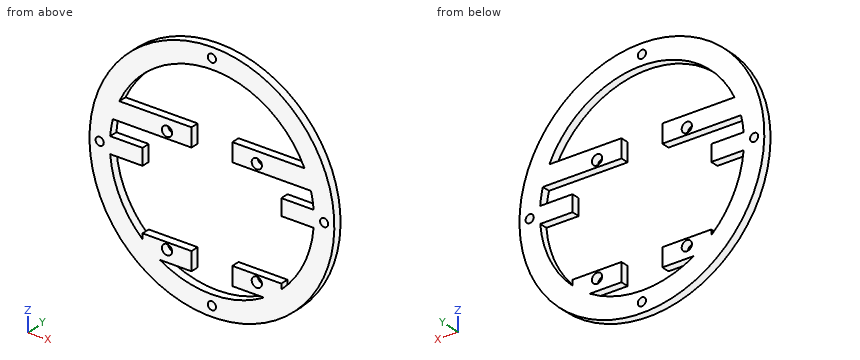
```python
from build123d import *

# Parameters (mm, degrees)
SKETCH1_R           = 30
SKETCH1_R_2         = 25
BOSS_EXTRUDE1_DEPTH = 2
SKETCH2_R           = 1
CUT_EXTRUDE1_DEPTH  = 43.473521163
BOSS_EXTRUDE2_DEPTH = 2
BOSS_EXTRUDE3_DEPTH = 2
CUT_EXTRUDE2_DEPTH  = 2
BOSS_EXTRUDE4_DEPTH = 2
SKETCH16_R          = 1.25
CUT_EXTRUDE3_DEPTH  = 2


with BuildPart() as part:
    # Sketch1 → Boss-Extrude1 (new body)
    with BuildSketch(Plane(origin=(0, 0, 0), x_dir=(1, 0, 0), z_dir=(0, 1, 0))):
        with Locations(Location((0, 0, 0), (0, 0, 270))):
            Circle(SKETCH1_R)
        with Locations(Location((0, 0, 0), (0, 0, 270))):
            Circle(SKETCH1_R_2, mode=Mode.SUBTRACT)
    extrude(amount=BOSS_EXTRUDE1_DEPTH)

    # Sketch2 → Cut-Extrude1 (cut, through all)
    with BuildSketch(Plane(origin=(0, 2, 0), x_dir=(1, 0, 0), z_dir=(0, 1, 0))):
        with Locations(Location((0, 27.5, 0), (0, 0, 270))):
            Circle(SKETCH2_R)
        with Locations(Location((27.5, 0, 0), (0, 0, 270))):
            Circle(SKETCH2_R)
        with Locations(Location((0, -27.5, 0), (0, 0, 270))):
            Circle(SKETCH2_R)
        with Locations(Location((-27.5, 0, 0), (0, 0, 270))):
            Circle(SKETCH2_R)
    extrude(amount=-CUT_EXTRUDE1_DEPTH, mode=Mode.SUBTRACT)

    # Sketch3 → Boss-Extrude2 (add)
    with BuildSketch(Plane(origin=(0, 0, 0), x_dir=(1, 0, 0), z_dir=(0, 1, 0))):
        with BuildLine():
            Line((-24.919871589, -2), (0, -2))
            Line((0, -2), (24.919871589, -2))
            ThreePointArc((24.919871589, -2), (25, 0), (24.919871589, 2))
            Line((24.919871589, 2), (-24.919871589, 2))
            ThreePointArc((-24.919871589, 2), (-25, 0), (-24.919871589, -2))
        make_face()
    extrude(amount=BOSS_EXTRUDE2_DEPTH)

    # Sketch13 → Boss-Extrude3 (add)
    with BuildSketch(Plane(origin=(0, 0, 0), x_dir=(1, 0, 0), z_dir=(0, 1, 0))):
        with BuildLine():
            Line((17, 0), (17, 18.33030278))
            ThreePointArc((17, 18.33030278), (14.962844887, 20.027812484), (12.757350822, 21.5))
            Line((12.757350822, 21.5), (5, 21.5))
            Line((5, 21.5), (5, -10.5))
            Line((5, -10.5), (17, -10.5))
            Line((17, -10.5), (17, 0))
        make_face()
        with BuildLine():
            Line((-5, 0), (-5, 21.5))
            Line((-5, 21.5), (-12.757350822, 21.5))
            ThreePointArc((-12.757350822, 21.5), (-14.962844887, 20.027812484), (-17, 18.33030278))
            Line((-17, 18.33030278), (-17, -10.5))
            Line((-17, -10.5), (-5, -10.5))
            Line((-5, -10.5), (-5, 0))
        make_face()
    extrude(amount=BOSS_EXTRUDE3_DEPTH)

    # Sketch14 → Cut-Extrude2 (cut)
    with BuildSketch(Plane(origin=(0, 2, 0), x_dir=(1, 0, 0), z_dir=(0, 1, 0))):
        Polygon((17, 0), (5, 0), (5, -2), (5, -6), (17, -6), (17, -2), align=None)
        Polygon((5, 2), (5, 0), (17, 0), (17, 2), (17, 17), (5, 17), align=None)
        Polygon((5, 0), (0, 0), (-5, 0), (-5, -2), (5, -2), align=None)
        Polygon((-5, 0), (0, 0), (5, 0), (5, 2), (-5, 2), align=None)
        Polygon((-17, 0), (-5, 0), (-5, 2), (-5, 17), (-17, 17), (-17, 2), align=None)
        Polygon((-5, -2), (-5, 0), (-17, 0), (-17, -2), (-17, -6), (-5, -6), align=None)
    extrude(amount=-CUT_EXTRUDE2_DEPTH, mode=Mode.SUBTRACT)


with BuildPart() as cut_extrude2_piece_1:
    # of the separate pieces the step leaves, piece 1, a body of its own (cut_extrude2_pieces)
    add(part.part.solids().sort_by_distance((0, 0, 30))[0])



with BuildPart() as cut_extrude2_piece_2:
    # of the separate pieces the step leaves, piece 2, a body of its own (cut_extrude2_pieces)
    add(part.part.solids().sort_by_distance((-17, 0, 6))[0])


with BuildPart() as cut_extrude2_piece_3:
    # of the separate pieces the step leaves, piece 3, a body of its own (cut_extrude2_pieces)
    add(part.part.solids().sort_by_distance((17, 0, 10.5))[0])


with BuildPart() as cut_extrude2_piece_1_1:
    add(cut_extrude2_piece_1.part)

    add(cut_extrude2_piece_2.part)  # Boss-Extrude4 merges Cut-Extrude2 piece 2

    add(cut_extrude2_piece_3.part)  # Boss-Extrude4 merges Cut-Extrude2 piece 3
    # Sketch15 → Boss-Extrude4 (add)
    with BuildSketch(Plane(origin=(0, 0, 0), x_dir=(1, 0, 0), z_dir=(0, 1, 0))):
        with BuildLine():
            Line((17, -6), (24.269322199, -6))
            ThreePointArc((24.269322199, -6), (23.586276437, -8.287796079), (22.688102609, -10.5))
            Line((22.688102609, -10.5), (17, -10.5))
            Line((17, -10.5), (17, -6))
        make_face()
        with BuildLine():
            Line((-17, -6), (-24.269322199, -6))
            ThreePointArc((-24.269322199, -6), (-23.586276437, -8.287796079), (-22.688102609, -10.5))
            Line((-22.688102609, -10.5), (-17, -10.5))
            Line((-17, -10.5), (-17, -6))
        make_face()
    extrude(amount=BOSS_EXTRUDE4_DEPTH)

    # Sketch16 → Cut-Extrude3 (cut)
    with BuildSketch(Plane(origin=(0, 2, 0), x_dir=(1, 0, 0), z_dir=(0, 1, 0))):
        with Locations(Location((11, 18.65, 0), (0, 0, 270))):
            Circle(SKETCH16_R)
        with Locations(Location((11, -7.65, 0), (0, 0, 270))):
            Circle(SKETCH16_R)
        with Locations(Location((-11, -7.65, 0), (0, 0, 270))):
            Circle(SKETCH16_R)
        with Locations(Location((-11, 18.65, 0), (0, 0, 270))):
            Circle(SKETCH16_R)
    extrude(amount=-CUT_EXTRUDE3_DEPTH, mode=Mode.SUBTRACT)


solid = cut_extrude2_piece_1_1.part
```
Work out the finished part from the listing and answer in its coordinate system (mm). Coordinates: 2 decimals unless noted, no trailing zeros. Write each loop counter-clockwise with the first axis right and the second up, starting at its lowest first coordinate (ties: lowest second). Pieces come first, ordered by that corner, then holes. Notation, with made-up numbers: (80.5, 79) - (117.5, 79) arc R36 ccw to (117.5, 114) - close; hole circle Ø2 at (2, 19). An arc over 180 degrees is marked (long way). Answer as a JSON object with one key per item and string values.
Q1. Find section B-B (x = 14). Write down the section's boundary in (y, z).
Results list:
{"outline": "(0, -26.53) - (2, -26.53) - (2, -17) - (0, -17) - close; (0, 6) - (2, 6) - (2, 10.5) - (0, 10.5) - close; (0, 20.71) - (2, 20.71) - (2, 26.53) - (0, 26.53) - close"}
Q2. Consider L1, parallel to X at y = 1, z = 0; L2, parallel to X at y = 0.4, z = -18.65; L3, parallel to Z at x = -22, y = 1.25. Determine where each line is inside the solid, lowest interval first. Write a range as from..to.
Results list:
{"L1": "x = -30..-28.5, -26.5..-17, 17..26.5, 28.5..30", "L2": "x = -23.5..-12.25, -9.75..-5, 5..9.75, 12.25..23.5", "L3": "z = -20.4..-11.87, -2..2, 6..10.5, 11.87..20.4"}
Q3. Find section D-D (x = -7.5). Write down the section's boundary in (y, z).
Results list:
{"outline": "(0, -29.05) - (2, -29.05) - (2, -23.85) - (0, -23.85) - close; (0, -21.5) - (2, -21.5) - (2, -17) - (0, -17) - close; (0, 6) - (2, 6) - (2, 10.5) - (0, 10.5) - close; (0, 23.85) - (2, 23.85) - (2, 29.05) - (0, 29.05) - close"}
Q4. Given pin 1 Ø0.6 at (y, z) = (1, 9) entering from -X; pin 2 Ø1 at (x, y) = (22, 1) entering from +Z; pin 3 Ø1 at (x, y) = (-10, 0.5) entering from +Z, each flat-ended and moving along its own axis, determine where each tip first touches the part or whether it passes through.
Results list:
{"pin 1": "stops at x = -28.71", "pin 2": "stops at z = 20.92", "pin 3": "stops at z = 28.46"}
Q5. Find section C-C (z = 0). Write down the section's boundary in (x, y), plus the area to 3 significant figures.
Results list:
{"outline": "(-30, 0) - (-28.5, 0) - (-28.5, 2) - (-30, 2) - close; (-26.5, 0) - (-17, 0) - (-17, 2) - (-26.5, 2) - close; (17, 0) - (26.5, 0) - (26.5, 2) - (17, 2) - close; (28.5, 0) - (30, 0) - (30, 2) - (28.5, 2) - close", "area": "44.0 mm^2"}
Q6. Find section A-A (z = 15). Write down the section's boundary in (x, y), plus the area to 3 significant figures.
Results list:
{"outline": "(-25.98, 0) - (-20, 0) - (-20, 2) - (-25.98, 2) - close; (20, 0) - (25.98, 0) - (25.98, 2) - (20, 2) - close", "area": "23.9 mm^2"}
